Work out the finished part from the listing and answer in its coordinate system (mm). A direction names the side the tool comes from. Coordinates: 2 decimals unless noted, no trailing zeros. Order: outer loops, then holes, each group sorted by start corner. A loop starts at its lowest first (then second) coordinate and runs counter-clockwise, first axis right, second up. Notation, with made-up numbers: M -39.5,65.25 L -26.5,65.25 A13 cw -26.5,72.25 Z; hole C 83.5,15.5 d7. An arc over 180 degrees is marked long. Use a Markdown table: item, result.
from build123d import *

# Parameters (mm, degrees)
F0_R      = 50.8
F1_DEPTH  = 38.1
F1_TAPER  = 35
F2_R      = 44.45
F3_DEPTH  = 31.75
F3_TAPER  = 35
F6_R      = 6.35
F13_W     = 40.0871150196
F13_H     = 221.6413393617
F14_DEPTH = 38.1
F16_R     = 63.4410735664
F17_DEPTH = 6.35
F17_TAPER = 45
F18_R     = 54.1198096159
F19_DEPTH = 3.175
F19_TAPER = 45
F20_R     = 2.38125
F21_DEPTH = 6.35
F23_W     = 544.7718501091
F23_H     = 283.927500248
F24_DEPTH = 65.204810909
F25_R     = 3.175
F26_DEPTH = 2.159


# Not quite as in the source:
# - a feature of the source that left no trace in its solid (it failed there, or was rolled back) is left out
# - a feature names something its author has since deleted; it is built from what else it names


with BuildPart() as f1:
    # F0 (on Top) → F1 (new body)
    with BuildSketch(Plane.XY):
        Circle(F0_R)
    extrude(amount=-F1_DEPTH, taper=F1_TAPER)

    # F2 (on face) → F3 (cut)
    with BuildSketch(Plane.XY):
        Circle(F2_R)
    extrude(amount=-F3_DEPTH, taper=F3_TAPER, mode=Mode.SUBTRACT)

    # F9: F7 across plane


with BuildPart() as f7:
    # F7: sweep along a path in F4
    with BuildLine(Plane.YZ) as f7_path:
        add(Plane.YZ * Edge.make_bspline(
            [(-50.8, 0), (-59.5457513783, -8.9993874064), (-82.8005315743, -30.8254243712), (-59.2938947205, -72.9983075974), (-50.8, -97.5854156721)],
            knots=[0, 0, 0, 0, 0.421582605, 1, 1, 1, 1], degree=3))
    # F6 (on plane+point) → F7 (sweep)
    with BuildSketch(Plane.XZ.offset(50.8)):
        with Locations((0, -6.35)):
            Circle(F6_R)
    sweep(path=f7_path.line)


with BuildPart() as f1_1:
    add(f1.part)
    add(f7.part.mirror(Plane.XZ))


with BuildPart() as f14_tool:
    # F13 (on plane+point) → F14 (new body)
    with BuildSketch(Plane.XY.offset(-103.303810809)):
        with Locations((2.3701563478, 10.5300284922)):
            Rectangle(F13_W, F13_H)
    extrude(amount=F14_DEPTH)


with BuildPart() as f1_2:
    add(f1_1.part)

    # F14: cut by f14_tool
    add(f14_tool.part, mode=Mode.SUBTRACT)



with BuildPart() as f7_1:
    add(f7.part)

    # F14: cut by f14_tool
    add(f14_tool.part, mode=Mode.SUBTRACT)


with BuildPart() as f1_3:
    add(f1_2.part)

    add(f7_1.part)  # F17 merges F7
    # F16 (on face) → F17 (join)
    with BuildSketch(Plane(origin=(0, 0, -65.203810809), x_dir=(1, 0, 0), z_dir=(0, 0, -1))):
        Circle(F16_R)
    extrude(amount=F17_DEPTH, taper=F17_TAPER)

    # F18 (on face) → F19 (cut)
    with BuildSketch(Plane.XY.offset(-65.203810809)):
        Circle(F18_R)
    extrude(amount=-F19_DEPTH, taper=F19_TAPER, mode=Mode.SUBTRACT)

    # F20 (on face) → F21 (cut, through all)
    with BuildSketch(Plane.XY.offset(-31.75)):
        Circle(F20_R)
    extrude(amount=-F21_DEPTH, mode=Mode.SUBTRACT)

    # F23 (on offset) → F24 (cut, through all)
    with BuildSketch(Plane.XY.offset(-65.203810809)):
        Rectangle(F23_W, F23_H)
    extrude(amount=F24_DEPTH, mode=Mode.SUBTRACT)

    # F25 (on face) → F26 (join)
    with BuildSketch(Plane.XY.offset(-65.203810809)):
        with Locations((0, 58.78068)):
            Circle(F25_R)
    f26 = extrude(amount=F26_DEPTH)

    # F27: F26 across plane
    add(f26.mirror(Plane.XZ))


solid = f1_3.part
(1) A cutting plane is placed at A-A (x = 0). Determine the outline of the cut face in (y, z), then the cut area to 3 significant figures.
Conclusion:
| item | result |
|---|---|
| outline | M -63.44,-65.2 L -57.09,-71.55 L 57.09,-71.55 L 63.44,-65.2 L 61.96,-65.2 L 61.96,-63.04 L 55.61,-63.04 L 55.61,-65.2 L 54.12,-65.2 L 50.94,-68.38 L -50.94,-68.38 L -54.12,-65.2 L -55.61,-65.2 L -55.61,-63.04 L -61.96,-63.04 L -61.96,-65.2 Z |
| area | 459 mm2 |
(2) Straight lines are drawn through the part: L1, parallel to Z at x = 26.5, y = 9; L2, parallel to X at y = -32, z = -66.25; L3, parallel to X at y = -16, z = -67.75. For each, find the intervals that lie inside material, in ascending order.
Conclusion:
| item | result |
|---|---|
| L1 | -71.55 to -68.38 |
| L2 | -53.56 to -42.34, 42.34 to 53.56 |
| L3 | -58.76 to -49.03, 49.03 to 58.76 |
(3) Determine the mould class of faces 1 (the conical face through (48.739, 15.349, -68.225)), 2 (the flat face through (0, -59, -63.045)), 3 (the cylindrical face through (-0.69, 55.68, -64.14)), 4 (the flat face through (-1, 1, -68.379)) for opening direction X: pulls with the +X half, pulls with the -X half, needs draft (parallel to the pull), parting line crosses it, or undercut.
Conclusion:
| item | result |
|---|---|
| face 1 | undercut |
| face 2 | needs draft |
| face 3 | parting line crosses it |
| face 4 | undercut |
(4) Which of the six approach directions +Z, -Z, +X, -X, +Y, -Y give full straight-line access (tool end or side, diameter ignored) to faces 5 (the flat face through (-1, -1, -71.554)), 6 (the cylindrical face through (-0.69, -55.68, -64.14))?
Conclusion:
| item | result |
|---|---|
| face 5 | -Z, +X, -X, +Y, -Y |
| face 6 | +Z |
(5) Given P1, Ø2, axis at x = -46, z = -69.5, coming from the +Y side; P2, Ø5, axis at y = -44.5, z = -65, coming from the +X side; P3, Ø5, axis at y = 47, z = -68.5, coming from the +X side, each flat-ended and moving along its own axis, determine where each tip first touches the part or whether it passes through.
Conclusion:
| item | result |
|---|---|
| P1 | y = 39.14 |
| P2 | x = 47.54 |
| P3 | x = 42.33 |
